Could you check a few things on this model? Use its own coordinates, in mm. A direction names the side the tool comes from. Give positions to 0.01 mm unless a question says otherwise; leave off trailing zeros. Write each loop counter-clockwise with the first axis right and the second up, starting at its lowest first coordinate (ties: lowest second). Pieces come first, ordered by that corner, then holes. Notation, with made-up numbers: (-31.5, 33.5) - (-5.5, 33.5) arc R19 cw to (-5.5, 47.5) - close; hole circle Ø5 at (-13, -13). An arc over 180 degrees is marked (long way). Write item = value, one per line.
from build123d import *

# Parameters (mm, degrees)
M8_CLEARANCE_HOLE1_D     = 9
M8_CLEARANCE_HOLE1_DEPTH = 15
CIRPATTERN1_COUNT        = 5


with BuildPart() as part:
    # Sketch2 → Revolve1 (revolve)
    with BuildSketch(Plane.XY):
        Polygon((-5, 11), (0, 11), (0, 30), (-5, 30), (-5, 60), (-20, 60), (-20, 40), (-10, 40), (-10, 12.5), (-20, 12.5), (-20, 8.5), (-5, 8.5), align=None)
    revolve(axis=Axis((-20, 0, 0), (1, 0, 0)))

    # M8 Clearance Hole1
    with Locations(Plane(origin=(-5, -50, 0), x_dir=(0, 0, 1), z_dir=(1, 0, 0))):
        with Locations((0, 0)):
            m8_clearance_hole1 = Hole(M8_CLEARANCE_HOLE1_D / 2, depth=M8_CLEARANCE_HOLE1_DEPTH)

    # CirPattern1: M8 Clearance Hole1 ×5 about axis
    cirpattern1_axis = Axis((0, 0, 0), (1, 0, 0))
    for i in range(1, CIRPATTERN1_COUNT):
        add(m8_clearance_hole1.rotate(cirpattern1_axis, i * 360 / CIRPATTERN1_COUNT), mode=Mode.SUBTRACT)


solid = part.part
1. If we section it at A-A, the plane y = 0: Please give me the cut outline in (x, z).
Filled sheet:
outline = (-20, -60) - (-5, -60) - (-5, -30) - (0, -30) - (0, -11) - (-5, -11) - (-5, -8.5) - (-20, -8.5) - (-20, -12.5) - (-10, -12.5) - (-10, -40) - (-20, -40) - close; (-20, 8.5) - (-5, 8.5) - (-5, 11) - (0, 11) - (0, 30) - (-5, 30) - (-5, 60) - (-20, 60) - (-20, 40) - (-10, 40) - (-10, 12.5) - (-20, 12.5) - close
2. If we section it at B-B, the plane z = 0: Please give me the cut outline in (x, y).
Filled sheet:
outline = (-20, -60) - (-5, -60) - (-5, -54.5) - (-20, -54.5) - close; (-20, -45.5) - (-5, -45.5) - (-5, -30) - (0, -30) - (0, -11) - (-5, -11) - (-5, -8.5) - (-20, -8.5) - (-20, -12.5) - (-10, -12.5) - (-10, -40) - (-20, -40) - close; (-20, 8.5) - (-5, 8.5) - (-5, 11) - (0, 11) - (0, 30) - (-5, 30) - (-5, 60) - (-20, 60) - (-20, 40) - (-10, 40) - (-10, 12.5) - (-20, 12.5) - close
3. Thinking about a two-plate mould opening in Z: for faces 1 (the face through (0, 0, -13)), 2 (the face through (-10, -9, 9)), 3 (the face through (-12.6, -59.94, 2.64)), 4 (the face through (-12.605, -11.786, -50.165)), which applies, pulls with the +Z half, pulls with the -Z half, needs draft (parallel to the pull), parting line crosses it, or undercut?
Filled sheet:
face_1 = needs draft
face_2 = undercut
face_3 = parting line crosses it
face_4 = undercut
4. I need wall thicknesses on line 1 (Z direction, x = -14.5, y = 0); line 2 (Y direction, x = -18, z = 33); line 3 (Y direction, x = -18.75, z = -32). Which ranges of each line are inside material? Lowest first, please.
Filled sheet:
line_1 = -60 to -40, -12.5 to -8.5, 8.5 to 12.5, 40 to 60
line_2 = -50.11 to -22.61, 22.61 to 37.77, 43.14 to 50.11
line_3 = -50.75 to -24, 24 to 36.79, 44.12 to 50.75
5. If we section it at D-D, the plane z = 38.5: Please give me the cut outline in (x, y).
Filled sheet:
outline = (-20, -46.02) - (-5, -46.02) - (-5, 46.02) - (-20, 46.02) - (-20, 10.85) - (-10, 10.85) - (-10, -10.85) - (-20, -10.85) - close
6. For pin 1 (5 mm diameter, centred on y = -28.5, z = 32, fed in from +X); pin 2 (6 mm diameter, centred on x = -4.5, z = 13.5, fed in from -Y); pin 3 (3 mm diameter, centred on y = -3.5, z = 26.5, fed in from -X), each with a flat end and sliding along its axis, tell me the tip position at first contact or that it passes through.
Filled sheet:
pin_1 = -5
pin_2 = -59.07
pin_3 = -10
7. If we section it at C-C, the plane x = -18.25: Count the separate pieces of the cut face and the enclosed holes in it, and give its area (3 significant figures).
Filled sheet:
separate_pieces = 2
enclosed_holes = 7
area = 6,230 mm2
8. Which directions (+Z, -Z, +X, -X, +Y, -Y) give clear straight access to the entire face, cutting with the end or side of a thin tool? Please do faces 5 (the face through (-5, -12, 28)), 6 (the face through (-12.6, 40.33, 24.89)), 7 (the face through (-14.93, -8.67, -39.05)).
Filled sheet:
face_5 = +X
face_6 = +X, -X
face_7 = -X
